Input: part model. Units: mm. Frame: model coordinates. A direction names the side the tool comes from. Coordinates: 2 decimals unless noted, no trailing zeros. Write each loop counter-clockwise with the first axis right and the second up, starting at its lowest first coordinate (ties: lowest second). Pieces come first, ordered by that corner, then holes. Notation, with made-up numbers: (57, -30) -> (63, -30) arc R20 ccw to (63, -18) -> close; hole circle Ø9 at (-29, 13.25). An arc over 180 degrees is marked (long way). One line per question, with ' | ' between items. Start each with the question number.
```python
from build123d import *

# Parameters (mm, degrees)
SKETCH1_R           = 7.5
BOSS_EXTRUDE1_DEPTH = 0.5
SKETCH3_R           = 8.5
SKETCH3_R_2         = 7
BOSS_EXTRUDE2_DEPTH = 0.5
BOSS_EXTRUDE3_START = 0.5
SKETCH4_R           = 8.5
SKETCH4_R_2         = 7
BOSS_EXTRUDE3_DEPTH = 0.5
SKETCH6_R           = 1.5
BOSS_EXTRUDE4_DEPTH = 45


with BuildPart() as part:
    # Sketch1 → Boss-Extrude1 (new, symmetric)
    with BuildSketch(Plane.XY):
        Circle(SKETCH1_R)
    extrude(amount=BOSS_EXTRUDE1_DEPTH, both=True)

    # Sketch3 → Boss-Extrude2 (add)
    with BuildSketch(Plane.XY.offset(0.5)):
        Circle(SKETCH3_R)
        Circle(SKETCH3_R_2, mode=Mode.SUBTRACT)
    extrude(amount=BOSS_EXTRUDE2_DEPTH)

    # Sketch4 → Boss-Extrude3 (add)
    with BuildSketch(Plane(origin=(0, 0, -0.5), x_dir=(-1, 0, 0), z_dir=(0, 0, -1)).offset(BOSS_EXTRUDE3_START)):
        with Locations(Location((0, 0, 0), (0, 0, 180))):
            Circle(SKETCH4_R)
        with Locations(Location((0, 0, 0), (0, 0, 180))):
            Circle(SKETCH4_R_2, mode=Mode.SUBTRACT)
    extrude(amount=-BOSS_EXTRUDE3_DEPTH)

    # Sketch6 → Boss-Extrude4 (add, symmetric)
    with BuildSketch(Plane.XY):
        with Locations(Location((0, 0, 0), (0, 0, 180))):
            Circle(SKETCH6_R)
    extrude(amount=BOSS_EXTRUDE4_DEPTH, both=True)


solid = part.part
```
1) Section D-D, the plane y = -5. Return loops of the section in (x, z).
2) Section A-A, the plane y = 0. Return loops of the section in (x, z), then the cut area to 3 significant figures.
3) First-contact query: P1, Ø1, axis at y = -2.5, z = -22.5, coming from the -X side; P2, Ø3, axis at x = 5.5, y = 2.5, coming from the +Z side; P3, Ø8, axis at y = 2.5, z = 25, coming from the +X side; P4, Ø5, axis at x = 1, y = 4, coming from the +Z side. Flat tips, straight axial feed; report the tip coordinate or a pass-through.
4) Access query for faces 1 (the face through (0, 2, 0.5)), 2 (the face through (-7.493, 0.33, 0.007)), 3 (the face through (-1.43, -0.45, -22.44)), 4 (the face through (0, 0, -45)). Directions: +Z, -Z, +X, -X, +Y, -Y. A direction counts if a zero-diameter tool reaches every point of the face in a straight line with its end or side. Return the directions, or none.
5) Section C-C, the plane z = 38. Return loops of the section in (x, y), then the cut area to 3 significant figures.
6) Ray query, line 1 (Y direction, x = 0, z = 0.65); line 2 (Z direction, x = 1.25, y = -7.5); line 3 (Z direction, x = 3.5, y = -6). Return the intervals inside material, ascending.
7) Pull-direction query (X, two-part tool) for faces 5 (the face through (0, 2, -0.5)), 6 (the face through (2, -7, -1)), 7 (the face through (6.466, 2.681, -0.754)), 8 (the face through (-1.107, -8.428, -0.754)); classes: released by +X, released by -X, zero draft, split by the parting line, or undercut.
Answer block:
1) outline: (-6.87, -1) -> (-4.9, -1) -> (-4.9, -0.5) -> (4.9, -0.5) -> (4.9, -1) -> (6.87, -1) -> (6.87, -0.5) -> (5.59, -0.5) -> (5.59, 0.5) -> (6.87, 0.5) -> (6.87, 1) -> (4.9, 1) -> (4.9, 0.5) -> (-4.9, 0.5) -> (-4.9, 1) -> (-6.87, 1) -> (-6.87, 0.5) -> (-5.59, 0.5) -> (-5.59, -0.5) -> (-6.87, -0.5) -> close
2) outline: (-8.5, -1) -> (-7, -1) -> (-7, -0.5) -> (-1.5, -0.5) -> (-1.5, -45) -> (1.5, -45) -> (1.5, -0.5) -> (7, -0.5) -> (7, -1) -> (8.5, -1) -> (8.5, -0.5) -> (7.5, -0.5) -> (7.5, 0.5) -> (8.5, 0.5) -> (8.5, 1) -> (7, 1) -> (7, 0.5) -> (1.5, 0.5) -> (1.5, 45) -> (-1.5, 45) -> (-1.5, 0.5) -> (-7, 0.5) -> (-7, 1) -> (-8.5, 1) -> (-8.5, 0.5) -> (-7.5, 0.5) -> (-7.5, -0.5) -> (-8.5, -0.5) -> close | area: 285 mm2
3) P1: passes through | P2: stops at z = 1 | P3: stops at x = 1.5 | P4: stops at z = 0.5
4) face 1: +Z | face 2: none | face 3: -Z | face 4: -Z, +X, -X, +Y, -Y
5) outline: circle Ø3 at (0, 0) | area: 7.07 mm2
6) line 1: y = -8.5 to -7, -1.5 to 1.5, 7 to 8.5 | line 2: z = -1 to -0.5, 0.5 to 1 | line 3: z = -0.5 to 0.5
7) face 5: undercut | face 6: zero draft | face 7: undercut | face 8: split by the parting line
